Design review of the part built by this model. Coordinates are the model's own, in mm. A direction names the side the tool comes from. Coordinates: 2 decimals unless noted, no trailing zeros. Write each loop counter-clockwise with the first axis right and the second up, starting at its lowest first coordinate (ties: lowest second). Pieces come first, ordered by that corner, then holes.
Q1. Take a section at A-A, the plane x = 0. Write out the cut boundary in (y, z), plus the area to 3 significant figures.
Q2. Take a section at C-C, the plane z = 0. Write out the cut boundary in (x, y), plus the area to 3 significant figures.
Q3. The part is to be moulded in two halves that separate along X. For faces 1 (the flat face through (0, 10, -15)), 2 (the cylindrical face through (2.994, 4.93, -22.804)), 3 (the cylindrical face through (10.758, 5.07, -16.806)), say which applies: released by +X, released by -X, zero draft, split by the parting line, or undercut.
Q4. Take a section at B-B, the plane y = 3. Write out the cut boundary in (x, z), plus the area to 3 significant figures.
Q5. Take a section at D-D, the plane z = 9. Write out the cut boundary in (x, y), plus the area to 3 significant figures.
Q6. For pin 1 Ø1 at (x, y) = (-5, 4) entering from +Z; pin 2 Ø1.5 at (x, y) = (15, 3.5) entering from -Z; pin 3 Ø2 at (x, y) = (-12.5, 8.5) entering from -Z, all flat-tipped, find the tip position at first contact; note any pin that passes through.
Q7. For L1, parallel to Z at x = 0, y = 1.1; L2, parallel to Z at x = 0, y = 4.5; L3, parallel to X at y = 7, z = 8, list the stretches that pass through material, from the lowest coordinate up.
Q8. For faces 4 (the cylindrical face through (-12.932, 5.944, 5.362)), 5 (the cylindrical face through (-20.186, 5.07, 0.221)), list the 3-axis set-ups (+Z, -Z, +X, -X, +Y, -Y) from which the entire face can be reached by the end or side of a thin tool; tool diameter is ignored.
Autodesk Inventor part; units mm, degrees
ref_plane "YZ Plane" through (0, 0, 0) normal (1, 0, 0) x (0, 1, 0)
ref_plane "XZ Plane" through (0, 0, 0) normal (0, 1, 0) x (-1, 0, 0)
ref_plane "XY Plane" through (0, 0, 0) normal (0, 0, 1) x (1, 0, 0)
sketch "Sketch1" plane through (0, 0, 0) normal (0, 1, 0) x (-1, 0, 0)
  circle A0 centre (0, 0) radius 14
  circle A1 centre (0, 0) radius 23
  line L0 (18.5, 0) -> (-9.25, -16.0215)
  line L1 (-9.25, -16.0215) -> (-9.25, 16.0215)
  line L2 (-9.25, 16.0215) -> (18.5, 0)
  circle A2 centre (0, 0) radius 12.5
  dimension "d0" = 28
  dimension "d1" = 46
  dimension "d2" = 18.5
  dimension "d3" = 25
extrude "Extrusion1" add sketch "Sketch1" along normal blind 10 contours A0 L2 L0 | A0 L1 L2 | L0 L1 A0 | A1
extrude "Extrusion2" add sketch "Sketch1" along normal blind 2 contours A0 L0 A2 L2 | L2 A2 A0 | A0 L0 A2 | L2 A2 L1 A0 | A0 L1 A2 L0 | L1 A2 A0
hole "Hole1" at (-18.5, 0, 0) at (9.25, 0, 16.0215) at (9.25, 0, -16.0215) direction (0, 1, 0) diameter 3.4 end through all
properties part number "cazoleta"
Responses:
1. outline: (0, -23) - (10, -23) - (10, -14) - (2, -14) - (2, -12.5) - (0, -12.5) - close; (0, 12.5) - (2, 12.5) - (2, 14) - (10, 14) - (10, 23) - (0, 23) - close
1. area: 186 mm2
2. outline: (-23, 0) - (-20.2, 0) - (-20.2, 10) - (-23, 10) - close; (-16.8, 0) - (-12.5, 0) - (-12.5, 2) - (-14, 2) - (-14, 10) - (-16.8, 10) - close; (12.5, 0) - (23, 0) - (23, 10) - (14, 10) - (14, 2) - (12.5, 2) - close
2. area: 152 mm2
3. face 1: zero draft
3. face 2: split by the parting line
3. face 3: undercut
4. outline: circle Ø46 at (0, 0); hole circle Ø3.4 at (-18.5, 0); hole circle Ø28 at (0, 0); hole circle Ø3.4 at (9.25, -16.02); hole circle Ø3.4 at (9.25, 16.02)
4. area: 1,020 mm2
5. outline: (-21.17, 0) - (-8.67, 0) - (-8.67, 2) - (-10.72, 2) - (-10.72, 10) - (-21.17, 10) - close; (8.67, 0) - (21.17, 0) - (21.17, 10) - (10.72, 10) - (10.72, 2) - (8.67, 2) - close
5. area: 217 mm2
6. pin 1: stops at z = 22.56
6. pin 2: stops at z = -18.05
6. pin 3: stops at z = -19.92
7. L1: z = -23 to -12.5, 12.5 to 23
7. L2: z = -23 to -14, 14 to 23
7. L3: x = -21.56 to -11.49, 11.49 to 21.56
8. face 4: +Y
8. face 5: +Y, -Y
